from build123d import *

# Parameters (mm, degrees)
BOSS_EXTRU_1_DEPTH           = 5
ESQUISSE11_R                 = 4.5
ENL_V_MAT_EXTRU_7_DEPTH      = 13
ENL_V_MAT_EXTRU_5_DEPTH      = 0.2
ESQUISSE2_R                  = 40.5
ENL_V_MAT_EXTRU_1_DEPTH      = 10
ESQUISSE3_R                  = 3
ENL_V_MAT_EXTRU_2_DEPTH      = 6
ESQUISSE10_R                 = 3.4
ENL_V_MAT_EXTRU_6_DEPTH      = 13
R_P_TITION_CIRCULAIRE1_COUNT = 4
BOSS_EXTRU_3_DEPTH           = 0.2
ESQUISSE26_W                 = 15
ESQUISSE26_H                 = 100
ENL_V_MAT_EXTRU_14_DEPTH     = 10
CONG_2_R                     = 10
ESQUISSE27_R                 = 2.5
ENL_V_MAT_EXTRU_15_DEPTH     = 10


with BuildPart() as part:
    # Esquisse1 → Boss.-Extru.1 (new body)
    with BuildSketch(Plane.XY):
        with BuildLine():
            Line((-98.507460241, 68.529411765), (-146.503153147, 68.529411765))
            Line((-146.503153147, 68.529411765), (-146.503153147, 168.529411765))
            Line((-146.503153147, 168.529411765), (-20.952657131, 168.529411765))
            ThreePointArc((-20.952657131, 168.529411765), (43.143624613, 155.983108662), (97.779066609, 120.196078431))
            ThreePointArc((97.779066609, 120.196078431), (129.667750386, -32.7851732), (0, -120))
            ThreePointArc((0, -120), (-84.852813742, -84.852813742), (-120, 0))
            ThreePointArc((-120, 0), (-114.500862942, 35.910338143), (-98.507460241, 68.529411765))
        make_face()
    extrude(amount=BOSS_EXTRU_1_DEPTH)

    # Esquisse11 → Enlèv. mat.-Extru.7 (cut)
    with BuildSketch(Plane.XY.offset(5)):
        with Locations((35.355339059, 35.355339059)):
            Circle(ESQUISSE11_R)
    enl_v_mat_extru_7 = extrude(amount=-ENL_V_MAT_EXTRU_7_DEPTH, mode=Mode.SUBTRACT)

    # Esquisse8 → Enlèv. mat.-Extru.5 (cut)
    with BuildSketch(Plane.XY.offset(5)):
        with BuildLine():
            Line((-148.503153147, 150.529411765), (-20.952657131, 150.529411765))
            ThreePointArc((-20.952657131, 150.529411765), (36.356959487, 139.311540755), (85.207472331, 107.31372549))
            ThreePointArc((85.207472331, 107.31372549), (112.996182479, -25.998508075), (0, -102))
            ThreePointArc((0, -102), (-98.056106388, -28.08914381), (-54.006119095, 86.529411765))
            Line((-54.006119095, 86.529411765), (-148.503153147, 86.529411765))
            Line((-148.503153147, 86.529411765), (-148.503153147, 150.529411765))
        make_face()
        with BuildLine():
            Line((-46.503153147, 88.529411765), (-146.503153147, 88.529411765))
            Line((-146.503153147, 88.529411765), (-146.503153147, 148.529411765))
            Line((-146.503153147, 148.529411765), (-20.952657131, 148.529411765))
            ThreePointArc((-20.952657131, 148.529411765), (35.602885584, 137.459144321), (83.810628522, 105.882352941))
            ThreePointArc((83.810628522, 105.882352941), (111.143786045, -25.244434172), (0, -100))
            ThreePointArc((0, -100), (-97.090012814, -23.948474101), (-46.503153147, 88.529411765))
        make_face(mode=Mode.SUBTRACT)
    extrude(amount=-ENL_V_MAT_EXTRU_5_DEPTH, mode=Mode.SUBTRACT)

    # Esquisse2 → Enlèv. mat.-Extru.1 (cut)
    with BuildSketch(Plane.XY.offset(5)):
        Circle(ESQUISSE2_R)
    extrude(amount=-ENL_V_MAT_EXTRU_1_DEPTH, mode=Mode.SUBTRACT)

    # Esquisse3 → Enlèv. mat.-Extru.2 (cut, through all)
    with BuildSketch(Plane(origin=(0, 0, 0), x_dir=(-1, 0, 0), z_dir=(0, 0, -1))):
        with Locations((16.656037964, 136.868437771)):
            Circle(ESQUISSE3_R)
    extrude(amount=-ENL_V_MAT_EXTRU_2_DEPTH, mode=Mode.SUBTRACT)

    # Esquisse10 → Enlèv. mat.-Extru.6 (cut)
    with BuildSketch(Plane.XY.offset(5)):
        with Locations((-121.503153147, 155.529411765)):
            Circle(ESQUISSE10_R)
        with Locations((117.617814583, 67.906676911)):
            Circle(ESQUISSE10_R)
        with Locations((100.297306508, -57.906676911)):
            Circle(ESQUISSE10_R)
        with Locations((0, -107)):
            Circle(ESQUISSE10_R)
        with Locations((-92.664718205, -53.5)):
            Circle(ESQUISSE10_R)
        with Locations((-92.664718205, 53.5)):
            Circle(ESQUISSE10_R)
        with Locations((-121.503153147, 81.529411765)):
            Circle(ESQUISSE10_R)
        with Locations((0, 154.124997046)):
            Circle(ESQUISSE10_R)
    extrude(amount=-ENL_V_MAT_EXTRU_6_DEPTH, mode=Mode.SUBTRACT)

    # Répétition circulaire1: Enlèv. mat.-Extru.7 ×4 about axis
    r_p_tition_circulaire1_axis = Axis((0, 0, 0), (0, 0, 1))
    for i in range(1, R_P_TITION_CIRCULAIRE1_COUNT):
        add(enl_v_mat_extru_7.rotate(r_p_tition_circulaire1_axis, i * 360 / R_P_TITION_CIRCULAIRE1_COUNT), mode=Mode.SUBTRACT)

    # Esquisse24 → Boss.-Extru.3 (add)
    with BuildSketch(Plane.XY.offset(5)):
        with BuildLine():
            Line((-146.503153147, 150.529411765), (-146.503153147, 148.529411765))
            Line((-146.503153147, 148.529411765), (-20.952657131, 148.529411765))
            ThreePointArc((-20.952657131, 148.529411765), (35.602885584, 137.459144321), (83.810628522, 105.882352941))
            ThreePointArc((83.810628522, 105.882352941), (111.143786045, -25.244434172), (0, -100))
            ThreePointArc((0, -100), (-97.090012814, -23.948474101), (-46.503153147, 88.529411765))
            Line((-46.503153147, 88.529411765), (-146.503153147, 88.529411765))
            Line((-146.503153147, 88.529411765), (-146.503153147, 86.529411765))
            Line((-146.503153147, 86.529411765), (-54.006119095, 86.529411765))
            ThreePointArc((-54.006119095, 86.529411765), (-98.056106388, -28.08914381), (0, -102))
            ThreePointArc((0, -102), (112.996182479, -25.998508075), (85.207472331, 107.31372549))
            ThreePointArc((85.207472331, 107.31372549), (36.356959487, 139.311540755), (-20.952657131, 150.529411765))
            Line((-20.952657131, 150.529411765), (-146.503153147, 150.529411765))
        make_face()
    extrude(amount=-BOSS_EXTRU_3_DEPTH)

    # Esquisse26 → Enlèv. mat.-Extru.14 (cut)
    with BuildSketch(Plane.XY.offset(5)):
        with Locations((-139.003153147, 118.529411765)):
            Rectangle(ESQUISSE26_W, ESQUISSE26_H)
    extrude(amount=-ENL_V_MAT_EXTRU_14_DEPTH, mode=Mode.SUBTRACT)

    # Congé2
    cong_2_edges = [part.edges().sort_by_distance(p)[0] for p in [
        (-131.503153147, 168.529411765, 2.5),
        (-131.503153147, 68.529411765, 2.5),
    ]]
    fillet(cong_2_edges, radius=CONG_2_R)

    # Esquisse27 → Enlèv. mat.-Extru.15 (cut)
    with BuildSketch(Plane.XY.offset(5)):
        with Locations((-116.503153147, 118.529411765)):
            Circle(ESQUISSE27_R)
        with Locations((0, 118.529411765)):
            Circle(ESQUISSE27_R)
        with Locations((66.701706035, 91.807022251)):
            Circle(ESQUISSE27_R)
        with Locations((85.55324371, -27.797933958)):
            Circle(ESQUISSE27_R)
        with Locations((0, -78)):
            Circle(ESQUISSE27_R)
        with Locations((-45.847249679, 63.103325561)):
            Circle(ESQUISSE27_R)
        with Locations((-78, 0)):
            Circle(ESQUISSE27_R)
    extrude(amount=-ENL_V_MAT_EXTRU_15_DEPTH, mode=Mode.SUBTRACT)


solid = part.part
Check sheet for the modelled part. Datum: model origin and axes. Units: mm. Round coordinates to 2 decimals unless told otherwise and drop trailing zeros. Loops run counter-clockwise (first coordinate to the right, second up) from the corner with the lowest first, then second, coordinate; pieces in that order, holes last.
1. Scan lines: probe 1 along Y at (x, z) = (0, 2.85) (3 decimals); probe 2 along Y at (x, z) = (-78, 1.2); probe 3 along X at (y, z) = (-26, 3.6). Record each from-to range of solid material in increasing order.
2. Sectioned sample at A-A on y = 53.5. Record the boundary of the cut face in (x, z).
3. Sectioned sample at D-D on y = 101. Record the boundary of the cut face in (x, z).
4. Sectioned sample at C-C on y = 10.5. Record the boundary of the cut face in (x, z).
5. Gauge pin test, flat end, axial feed: pin 1 Ø4.5 at (x, y) = (0, 118.53) entering from -Z. Record the tip position at first contact, or that the pin passes through.
6. Sectioned sample at B-B on z = 2.5. Give the number of separate pieces and of enclosed holes in the cut face, and give its area (3 significant figures).
7. Mould release check, pull along Y, two halves, no side actions. Record for faces 1 (the flat face through (6, 58, 0)), 2 (the cylindrical face through (42.29, 156.33, 2.46)), 3 (the cylindrical face through (-2.506, -104.702, 2.535)): released by +Y, released by -Y, zero draft, split by the parting line, or undercut.
Recorded:
1. probe 1: y = -120 to -110.4, -103.6 to -80.5, -75.5 to -40.5, 40.5 to 116.029, 121.029 to 150.725, 157.525 to 167.233
1. probe 2: y = -91.19 to -2.5, 2.5 to 168.53
1. probe 3: x = -117.15 to -31.05, 31.05 to 83.82, 87.29 to 132.23
2. outline: (-107.41, 0) - (-96.06, 0) - (-96.06, 5) - (-107.41, 5) - close; (-89.26, 0) - (135.93, 0) - (135.93, 5) - (-89.26, 5) - close
3. outline: (-131.5, 0) - (114.19, 0) - (114.19, 5) - (-131.5, 5) - close
4. outline: (-119.54, 0) - (-39.12, 0) - (-39.12, 5) - (-119.54, 5) - close; (39.12, 0) - (139.68, 0) - (139.68, 5) - (39.12, 5) - close
5. pin 1: passes through
6. separate pieces: 1
6. enclosed holes: 21
6. area: 57,400 mm2
7. face 1: zero draft
7. face 2: released by +Y
7. face 3: undercut
